Build history of the part. All positions in model axes, mm. A direction names the side the tool comes from. Round coordinates to 2 decimals unless told otherwise and drop trailing zeros. Write each loop counter-clockwise with the first axis right and the second up, starting at its lowest first coordinate (ties: lowest second). Pieces come first, ordered by that corner, then holes. Notation, with made-up numbers: (17.5, 27) -> (25.5, 27) arc R5 cw to (25.5, 31) -> close; hole circle Ø11 at (34.25, -36.75). An arc over 180 degrees is marked (long way). Return JSON: item names as keys, results as strings.
from build123d import *

# Parameters (mm, degrees)
SKETCH_1_R          = 2
EXTRUDE_1_DEPTH     = 16
SKETCH_2_R          = 3.52854217
EXTRUDE_3_DEPTH     = 3
CUT_EXTRUDE_2_DEPTH = 1.5
CHAMFER_1_SIZE      = 0.2
CHAMFER_2_SIZE      = 0.2


with BuildPart() as part:
    # 草图1 → 凸台-拉伸1 (new body)
    with BuildSketch(Plane.XY):
        Circle(SKETCH_1_R)
    extrude(amount=EXTRUDE_1_DEPTH)

    # 草图2 → 凸台-拉伸3 (add)
    with BuildSketch(Plane.XY.offset(16)):
        Circle(SKETCH_2_R)
    extrude(amount=EXTRUDE_3_DEPTH)

    # 草图3 → 切除-拉伸2 (cut)
    with BuildSketch(Plane.XY.offset(19)):
        Polygon((0, 2.497687594), (-2.163060907, 1.248843797), (-2.163060907, -1.248843797), (0, -2.497687594), (2.163060907, -1.248843797), (2.163060907, 1.248843797), align=None)
    extrude(amount=-CUT_EXTRUDE_2_DEPTH, mode=Mode.SUBTRACT)

    # 倒角1
    chamfer_1_edges = [part.edges().sort_by_distance(p)[0] for p in [
        (-2, 0, 0),
    ]]
    chamfer(chamfer_1_edges, length=CHAMFER_1_SIZE)

    # 倒角2
    chamfer_2_edges = [part.edges().sort_by_distance(p)[0] for p in [
        (-3.52854217, 0, 16),
        (-3.52854217, 0, 19),
    ]]
    chamfer(chamfer_2_edges, length=CHAMFER_2_SIZE)


solid = part.part
Q1. Wall check: L1, parallel to Z at x = 2, y = 2.5; L2, parallel to Z at x = 0.75, y = 2; L3, parallel to X at y = -0.75, z = 5. Give the ranges that are in metal, low to high.
Verdict:
{"L1": "z = 16 to 19", "L2": "z = 16 to 17.5", "L3": "x = -1.85 to 1.85"}
Q2. Saw through at B-B on z = 10. List the corners of the cut face in (x, y), then the cut area to 3 significant figures.
Verdict:
{"outline": "circle Ø4 at (0, 0)", "area": "12.6 mm²"}
Q3. 3-axis set-ups, long thin cutter, end or side, ignore diameter. For faces 4 (the cylindrical face through (0, -2, 8)), 5 (the flat face through (0, 0, 0)), 6 (the flat face through (-1.07, 1.88, 18.26)): which of +Z, -Z, +X, -X, +Y, -Y reach the whole face in a straight line?
Verdict:
{"face 4": "-Z", "face 5": "-Z, +X, -X, +Y, -Y", "face 6": "+Z"}
Q4. Pin check, flat tips, straight feed: pin 1 Ø1.5 at (y, z) = (-0.5, 15.5) entering from +X; pin 2 Ø1.5 at (y, z) = (-0.5, 8) entering from -X; pin 3 Ø1.3 at (x, y) = (0.5, 1) entering from +Z. Stop position of each tip, or through.
Verdict:
{"pin 1": "stops at x = 3.52", "pin 2": "stops at x = -2", "pin 3": "stops at z = 17.5"}
Q5. Two-plate mould, pull along Y, no slides. Class faces 1 (the cylindrical face through (-0.46, 3.5, 17.48)), 2 (the flat face through (-2.163, 0, 18)), 3 (the flat face through (0, -2.2, 16)): +Y half, -Y half, draft (parallel to the pull), parting line (faces both ways), or undercut.
Verdict:
{"face 1": "parting line", "face 2": "undercut", "face 3": "draft"}
Q6. Saw through at A-A on y = 0. List the corners of the cut face in (x, z).
Verdict:
{"outline": "(-3.53, 16.2) -> (-3.33, 16) -> (-2, 16) -> (-2, 0.2) -> (-1.8, 0) -> (1.8, 0) -> (2, 0.2) -> (2, 16) -> (3.33, 16) -> (3.53, 16.2) -> (3.53, 18.8) -> (3.33, 19) -> (2.16, 19) -> (2.16, 17.5) -> (-2.16, 17.5) -> (-2.16, 19) -> (-3.33, 19) -> (-3.53, 18.8) -> close"}
